from build123d import *

# Parameters (mm, degrees)
BOSS_EXTRUDE1_DEPTH          = 6.35
SKETCH2_R                    = 4
CUT_EXTRUDE1_DEPTH           = 1.5875
SKETCH3_R                    = 1.190625
CUT_EXTRUDE2_DEPTH           = 6.35
CIRPATTERN1_COUNT            = 4
CIRPATTERN2_COPY_1_SKETCH_R  = 1.190625
CIRPATTERN2_COPY_1_DEPTH     = 6.35
CIRPATTERN2_COPY_2_SKETCH_R  = 1.190625
CIRPATTERN2_COPY_2_DEPTH     = 6.35
CIRPATTERN2_COPY_3_SKETCH_R  = 1.190625
CIRPATTERN2_COPY_3_DEPTH     = 6.35
CIRPATTERN2_COPY_4_SKETCH_R  = 1.190625
CIRPATTERN2_COPY_4_DEPTH     = 6.35
CIRPATTERN2_COPY_5_SKETCH_R  = 1.190625
CIRPATTERN2_COPY_5_DEPTH     = 6.35
CIRPATTERN2_COPY_6_SKETCH_R  = 1.190625
CIRPATTERN2_COPY_6_DEPTH     = 6.35
CIRPATTERN2_COPY_7_SKETCH_R  = 1.190625
CIRPATTERN2_COPY_7_DEPTH     = 6.35
CIRPATTERN2_COPY_8_SKETCH_R  = 1.190625
CIRPATTERN2_COPY_8_DEPTH     = 6.35
CIRPATTERN2_COPY_9_SKETCH_R  = 1.190625
CIRPATTERN2_COPY_9_DEPTH     = 6.35
CIRPATTERN2_COPY_10_SKETCH_R = 1.190625
CIRPATTERN2_COPY_10_DEPTH    = 6.35
CIRPATTERN2_COPY_11_SKETCH_R = 1.190625
CIRPATTERN2_COPY_11_DEPTH    = 6.35
CIRPATTERN2_COPY_12_SKETCH_R = 1.190625
CIRPATTERN2_COPY_12_DEPTH    = 6.35


with BuildPart() as part:
    # Sketch1 → Boss-Extrude1 (new body)
    with BuildSketch(Plane.XY):
        with BuildLine():
            Line((-12.7, -76.2), (-12.7, 76.2))
            ThreePointArc((-12.7, 76.2), (0, 88.9), (12.7, 76.2))
            Line((12.7, 76.2), (12.7, -76.2))
            ThreePointArc((12.7, -76.2), (0, -88.9), (-12.7, -76.2))
        make_face()
    extrude(amount=BOSS_EXTRUDE1_DEPTH)

    # Sketch2 → Cut-Extrude1 (cut)
    with BuildSketch(Plane.XY.offset(6.35)):
        with Locations((0, 76.2)):
            Circle(SKETCH2_R)
    cut_extrude1 = extrude(amount=-CUT_EXTRUDE1_DEPTH, mode=Mode.SUBTRACT)

    # Mirror1: Cut-Extrude1 across plane
    add(cut_extrude1.mirror(Plane.ZX), mode=Mode.SUBTRACT)

    # Sketch3 → Cut-Extrude2 (cut)
    with BuildSketch(Plane.XY.offset(6.35)):
        with Locations((0, 83.2)):
            Circle(SKETCH3_R)
        with Locations((0, -69.2)):
            Circle(SKETCH3_R)
    cut_extrude2 = extrude(amount=-CUT_EXTRUDE2_DEPTH, mode=Mode.SUBTRACT)

    # CirPattern1: Cut-Extrude2 ×4 about axis
    cirpattern1_axis = Axis((0, 76.2, 0), (0, 0, 1))
    for i in range(1, CIRPATTERN1_COUNT):
        add(cut_extrude2.rotate(cirpattern1_axis, i * 360 / CIRPATTERN1_COUNT), mode=Mode.SUBTRACT)

    # CirPattern2 copy 1 sketch → CirPattern2 copy 1 (cut)
    with BuildSketch(Plane(origin=(-152.4, 0, 6.35), x_dir=(-1, 0, 0), z_dir=(0, 0, 1))):
        with Locations((0, 83.2)):
            Circle(CIRPATTERN2_COPY_1_SKETCH_R)
        with Locations((0, -69.2)):
            Circle(CIRPATTERN2_COPY_1_SKETCH_R)
    extrude(amount=-CIRPATTERN2_COPY_1_DEPTH, mode=Mode.SUBTRACT)

    # CirPattern2 copy 2 sketch → CirPattern2 copy 2 (cut)
    with BuildSketch(Plane(origin=(-76.2, -228.6, 6.35), x_dir=(0, -1, 0), z_dir=(0, 0, 1))):
        with Locations((0, 83.2)):
            Circle(CIRPATTERN2_COPY_2_SKETCH_R)
        with Locations((0, -69.2)):
            Circle(CIRPATTERN2_COPY_2_SKETCH_R)
    extrude(amount=-CIRPATTERN2_COPY_2_DEPTH, mode=Mode.SUBTRACT)

    # CirPattern2 copy 3 sketch → CirPattern2 copy 3 (cut)
    with BuildSketch(Plane(origin=(152.4, -152.4, 6.35), x_dir=(1, 0, 0), z_dir=(0, 0, 1))):
        with Locations((0, 83.2)):
            Circle(CIRPATTERN2_COPY_3_SKETCH_R)
        with Locations((0, -69.2)):
            Circle(CIRPATTERN2_COPY_3_SKETCH_R)
    extrude(amount=-CIRPATTERN2_COPY_3_DEPTH, mode=Mode.SUBTRACT)

    # CirPattern2 copy 4 sketch → CirPattern2 copy 4 (cut)
    with BuildSketch(Plane(origin=(-228.6, -76.2, 6.35), x_dir=(0, -1, 0), z_dir=(0, 0, 1))):
        with Locations((0, 83.2)):
            Circle(CIRPATTERN2_COPY_4_SKETCH_R)
        with Locations((0, -69.2)):
            Circle(CIRPATTERN2_COPY_4_SKETCH_R)
    extrude(amount=-CIRPATTERN2_COPY_4_DEPTH, mode=Mode.SUBTRACT)

    # CirPattern2 copy 5 sketch → CirPattern2 copy 5 (cut)
    with BuildSketch(Plane(origin=(0, -304.8, 6.35), x_dir=(1, 0, 0), z_dir=(0, 0, 1))):
        with Locations((0, 83.2)):
            Circle(CIRPATTERN2_COPY_5_SKETCH_R)
        with Locations((0, -69.2)):
            Circle(CIRPATTERN2_COPY_5_SKETCH_R)
    extrude(amount=-CIRPATTERN2_COPY_5_DEPTH, mode=Mode.SUBTRACT)

    # CirPattern2 copy 6 sketch → CirPattern2 copy 6 (cut)
    with BuildSketch(Plane(origin=(228.6, -76.2, 6.35), x_dir=(0, 1, 0), z_dir=(0, 0, 1))):
        with Locations((0, 83.2)):
            Circle(CIRPATTERN2_COPY_6_SKETCH_R)
        with Locations((0, -69.2)):
            Circle(CIRPATTERN2_COPY_6_SKETCH_R)
    extrude(amount=-CIRPATTERN2_COPY_6_DEPTH, mode=Mode.SUBTRACT)

    # CirPattern2 copy 7 sketch → CirPattern2 copy 7 (cut)
    with BuildSketch(Plane(origin=(-152.4, -152.4, 6.35), x_dir=(1, 0, 0), z_dir=(0, 0, 1))):
        with Locations((0, 83.2)):
            Circle(CIRPATTERN2_COPY_7_SKETCH_R)
        with Locations((0, -69.2)):
            Circle(CIRPATTERN2_COPY_7_SKETCH_R)
    extrude(amount=-CIRPATTERN2_COPY_7_DEPTH, mode=Mode.SUBTRACT)

    # CirPattern2 copy 8 sketch → CirPattern2 copy 8 (cut)
    with BuildSketch(Plane(origin=(76.2, -228.6, 6.35), x_dir=(0, 1, 0), z_dir=(0, 0, 1))):
        with Locations((0, 83.2)):
            Circle(CIRPATTERN2_COPY_8_SKETCH_R)
        with Locations((0, -69.2)):
            Circle(CIRPATTERN2_COPY_8_SKETCH_R)
    extrude(amount=-CIRPATTERN2_COPY_8_DEPTH, mode=Mode.SUBTRACT)

    # CirPattern2 copy 9 sketch → CirPattern2 copy 9 (cut)
    with BuildSketch(Plane(origin=(152.4, 0, 6.35), x_dir=(-1, 0, 0), z_dir=(0, 0, 1))):
        with Locations((0, 83.2)):
            Circle(CIRPATTERN2_COPY_9_SKETCH_R)
        with Locations((0, -69.2)):
            Circle(CIRPATTERN2_COPY_9_SKETCH_R)
    extrude(amount=-CIRPATTERN2_COPY_9_DEPTH, mode=Mode.SUBTRACT)

    # CirPattern2 copy 10 sketch → CirPattern2 copy 10 (cut)
    with BuildSketch(Plane(origin=(-76.2, -76.2, 6.35), x_dir=(0, 1, 0), z_dir=(0, 0, 1))):
        with Locations((0, 83.2)):
            Circle(CIRPATTERN2_COPY_10_SKETCH_R)
        with Locations((0, -69.2)):
            Circle(CIRPATTERN2_COPY_10_SKETCH_R)
    extrude(amount=-CIRPATTERN2_COPY_10_DEPTH, mode=Mode.SUBTRACT)

    # CirPattern2 copy 11 sketch → CirPattern2 copy 11 (cut)
    with BuildSketch(Plane(origin=(0, -152.4, 6.35), x_dir=(-1, 0, 0), z_dir=(0, 0, 1))):
        with Locations((0, 83.2)):
            Circle(CIRPATTERN2_COPY_11_SKETCH_R)
        with Locations((0, -69.2)):
            Circle(CIRPATTERN2_COPY_11_SKETCH_R)
    extrude(amount=-CIRPATTERN2_COPY_11_DEPTH, mode=Mode.SUBTRACT)

    # CirPattern2 copy 12 sketch → CirPattern2 copy 12 (cut)
    with BuildSketch(Plane(origin=(76.2, -76.2, 6.35), x_dir=(0, -1, 0), z_dir=(0, 0, 1))):
        with Locations((0, 83.2)):
            Circle(CIRPATTERN2_COPY_12_SKETCH_R)
        with Locations((0, -69.2)):
            Circle(CIRPATTERN2_COPY_12_SKETCH_R)
    extrude(amount=-CIRPATTERN2_COPY_12_DEPTH, mode=Mode.SUBTRACT)


solid = part.part
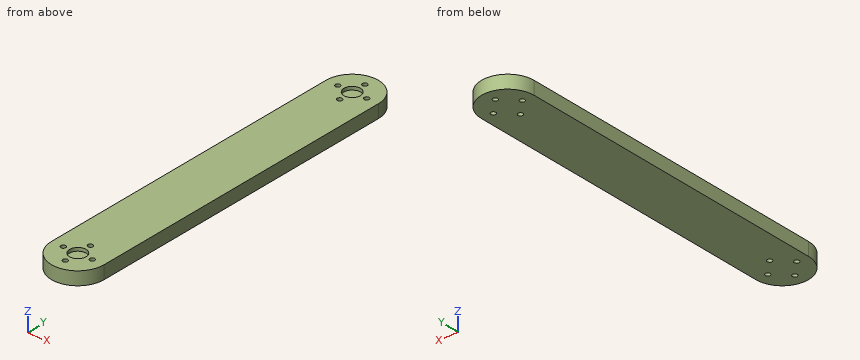
Geometry check sheet. Reference: the model listing, model coordinates, mm. Round coordinates to 2 decimals unless told otherwise and drop trailing zeros. Order: outer loops, then holes, each group sorted by start corner. A loop starts at its lowest first (then second) coordinate and runs counter-clockwise, first axis right, second up. Notation, with made-up numbers: M 63.25,83.5 L 75.25,83.5 A8 cw 75.25,93.5 Z; hole C 79.5,-7.5 d3. An arc over 180 degrees is marked long. Answer in a Markdown table with one row per item. Add a question column.
Item 1: Material ranges on L1, parallel to X at y = -76.2, z = 3; L2, parallel to Y at x = 0, z = 2.25; L3, parallel to X at y = -69.2, z = 5, recorded low to high. Write a range as [from, to].
Item 2: Sectioned sample at B-B, the plane x = -10.25. Enter the section's corners in (y, z), plus the area to 3 significant figures.
Item 3: Depth check by flat-ended pin: pin 1 Ø2.5 at (x, y) = (0, -69.2) entering from -Z; pin 2 Ø6.5 at (x, y) = (0, 76.2) entering from +Z; pin 3 Ø1 at (x, z) = (10, 3.5) entering from +Y; pin 4 Ø1.4 at (x, y) = (-7, -76.2) entering from +Z. Enter the tip coordinate at first touch or a pass-through.
Item 4: Sectioned sample at A-A, the plane z = 2.5. State how many separate pieces and enclosed holes the cut face has, plus the area to 3 significant figures.
Filled in:
| question | item | result |
|---|---|---|
| 1 | L1 | x = [-12.7, -8.19], [-5.81, 5.81], [8.19, 12.7] |
| 1 | L2 | y = [-88.9, -84.39], [-82.01, -70.39], [-68.01, 68.01], [70.39, 82.01], [84.39, 88.9] |
| 1 | L3 | x = [-12.7, -1.19], [1.19, 12.7] |
| 2 | outline | M -83.7,0 L 83.7,0 L 83.7,6.35 L -83.7,6.35 Z |
| 2 | area | 1,060 mm² |
| 3 | pin 1 | stops at z = 0 |
| 3 | pin 2 | stops at z = 4.76 |
| 3 | pin 3 | stops at y = 84.63 |
| 3 | pin 4 | passes through |
| 4 | separate pieces | 1 |
| 4 | enclosed holes | 8 |
| 4 | area | 4,340 mm² |
